Work out the finished part from the listing and answer in its coordinate system (mm). Face numbers are marked on the shaded views. Give positions to 0.01 mm unless a question says otherwise; leave off trailing zeros. Loops run counter-clockwise (first coordinate to the right, second up) from the corner with the lowest first, then second, coordinate; pieces in that order, holes last. Notation, with made-up numbers: M 38,66 L 96,66 A11 ccw 96,80 Z; hole C 5.5,-3 d2. An arc over 180 degrees is marked long. Write item = value, one per line. Start each with the question number.
1. A flat-ended cylindrical pin translates along its axis: pin 1 Ø1 at (y, z) = (3.5, 1.5) entering from +X. Find the tip coordinate at first contact, or state that the pin passes through.
2. Section D-D on x = -28 is taken. Determine the outline of the cut face in (y, z), plus the area to 3 significant figures.
3. Consider L1, parallel to Y at x = -1, z = 1.45; L2, parallel to X at y = 6.25, z = 0.2; L3, parallel to Y at x = -29.5, z = 1. Determine where each line is inside the solid, lowest interval first. Write a range as [from, to].
4. The mould has two halves that part along Y. Classify the marked faces 1, 2 and 3: released by +Y, released by -Y, zero draft, split by the parting line, or undercut.
5. Section B-B on z = 0.5 is taken. Determine the outline of the cut face in (x, y), plus the area to 3 significant figures.
6. Section A-A on x = -0.5 is taken. Determine the outline of the cut face in (y, z).
7. Section C-C on y = 7.75 is taken. Determine the outline of the cut face in (x, z).
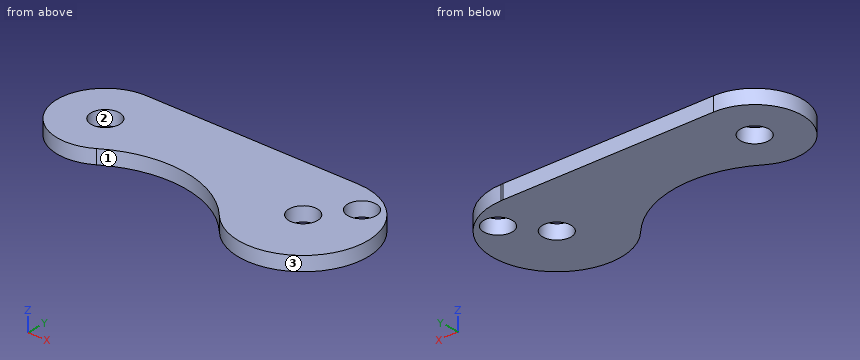
```python
from build123d import *

# Parameters (mm, degrees)
SKETCH1_R           = 2
BOSS_EXTRUDE1_DEPTH = 2


with BuildPart() as part:
    # Sketch1 → Boss-Extrude1 (new body)
    with BuildSketch(Plane.XY):
        with BuildLine():
            Line((-1.2887257, 9.27170727), (-31.0207003, 8.828891045))
            ThreePointArc((-31.0207003, 8.828891045), (-37.4360697, 0.196784564), (-27.320647525, -3.456770014))
            ThreePointArc((-27.320647525, -3.456770014), (-17.039618289, -1.022120458), (-7.632023625, -5.830887792))
            ThreePointArc((-7.632023625, -5.830887792), (7.224276423, -3.332674299), (-1.0207003, 9.275699134))
            Line((-1.0207003, 9.275699134), (-1.2887257, 9.27170727))
        make_face()
        with Locations((-31.0207003, 2.128891045)):
            Circle(SKETCH1_R, mode=Mode.SUBTRACT)
        with Locations((-1.0207003, 0.275699134)):
            Circle(SKETCH1_R, mode=Mode.SUBTRACT)
        with Locations((2.9792997, 5.275699134)):
            Circle(SKETCH1_R, mode=Mode.SUBTRACT)
    extrude(amount=BOSS_EXTRUDE1_DEPTH)


solid = part.part
```
Verdict:
q1.pin_1 = 7.56
q2.outline = M -3.85,0 L 8.87,0 L 8.87,2 L -3.85,2 Z
q2.area = 25.5 mm2
q3.L1 = [-8.72, -1.72], [2.28, 9.28]
q3.L2 = [-36.3, 1.23], [4.73, 5.71]
q3.L3 = [-4.4, 0.83], [3.43, 8.85]
q4.face_1 = released by -Y
q4.face_2 = undercut
q4.face_3 = split by the parting line
q5.outline = M -31.02,8.83 A6.7 ccw long -27.32,-3.46 A15.3 cw -7.63,-5.83 A9 ccw long -1.02,9.28 Z; hole C -31.02,2.13 d4; hole C -1.02,0.28 d4; hole C 2.98,5.28 d4
q5.area = 541 mm2
q6.outline = M -8.71,0 L -1.66,0 L -1.66,2 L -8.71,2 Z; M 2.21,0 L 9.26,0 L 9.26,2 L 2.21,2 Z
q7.outline = M -34.67,0 L 3.99,0 L 3.99,2 L -34.67,2 Z
